```python
from build123d import *

# Parameters (mm, degrees)
SKETCH1_W                = 130
SKETCH1_H                = 80
BOSS_EXTRUDE1_DEPTH      = 2
CUT_EXTRUDE_THIN1_DEPTH  = 3.2
BOSS_EXTRUDE2_DEPTH      = 10
BOSS_EXTRUDE2_DEPTH_BACK = 15
SKETCH5_R                = 1.5
BOSS_EXTRUDE3_DEPTH      = 10
BOSS_EXTRUDE3_DEPTH_BACK = 12
SKETCH6_R                = 2
SKETCH9_W                = 5
SKETCH9_H                = 50
BOSS_EXTRUDE5_DEPTH      = 10.5
SKETCH11_R               = 1.5
CUT_EXTRUDE1_DEPTH       = 7.5


with BuildPart() as part:
    # Sketch1 → Boss-Extrude1 (new body)
    with BuildSketch(Plane.XY):
        with Locations((65, 40)):
            Rectangle(SKETCH1_W, SKETCH1_H)
    extrude(amount=BOSS_EXTRUDE1_DEPTH)

    # Sketch2 → Cut-Extrude-Thin1 (cut)
    with BuildSketch(Plane.XY.offset(2)):
        with BuildLine():
            Line((49.817075189, 61.102777477), (79.817075189, 57.949650419))
            ThreePointArc((79.817075189, 57.949650419), (81.8288026, 55.594220253), (79.581886147, 53.461976154))
            Line((79.581886147, 53.461976154), (49.581886147, 53.461976154))
            ThreePointArc((49.581886147, 53.461976154), (43.839766322, 48.012907902), (48.980847483, 41.993475256))
            Line((48.980847483, 41.993475256), (68.980847483, 39.89139055))
            ThreePointArc((68.980847483, 39.89139055), (70.992574894, 37.535960384), (68.745658441, 35.403716286))
            Line((68.745658441, 35.403716286), (48.745658441, 35.403716286))
            ThreePointArc((48.745658441, 35.403716286), (43.003538616, 29.954648034), (48.144619777, 23.935215387))
            Line((48.144619777, 23.935215387), (102.144619777, 18.259586683))
            Line((102.144619777, 18.259586683), (102.510469398, 21.740413317))
            Line((102.510469398, 21.740413317), (48.510469398, 27.416042021))
            ThreePointArc((48.510469398, 27.416042021), (46.498741988, 29.771472187), (48.745658441, 31.903716286))
            Line((48.745658441, 31.903716286), (68.745658441, 31.903716286))
            ThreePointArc((68.745658441, 31.903716286), (74.487778266, 37.352784537), (69.346697105, 43.372217184))
            Line((69.346697105, 43.372217184), (49.346697105, 45.47430189))
            ThreePointArc((49.346697105, 45.47430189), (47.334969694, 47.829732056), (49.581886147, 49.961976154))
            Line((49.581886147, 49.961976154), (79.581886147, 49.961976154))
            ThreePointArc((79.581886147, 49.961976154), (85.324005972, 55.411044406), (80.182924811, 61.430477052))
            Line((80.182924811, 61.430477052), (50.182924811, 64.58360411))
            Line((50.182924811, 64.58360411), (49.817075189, 61.102777477))
        make_face()
    extrude(amount=-CUT_EXTRUDE_THIN1_DEPTH, mode=Mode.SUBTRACT)

    # Sketch5 → Boss-Extrude2 (add, two sides: drawn at the far end of the back side and taken through both)
    with BuildSketch(Plane(origin=(0, 0, 0), x_dir=(-1, 0, 0), z_dir=(0, 0, -1)).offset(-BOSS_EXTRUDE2_DEPTH_BACK)):
        with Locations((-115, 10)):
            Circle(SKETCH5_R)
    extrude(amount=BOSS_EXTRUDE2_DEPTH + BOSS_EXTRUDE2_DEPTH_BACK)

    # Sketch6 → Boss-Extrude3 (add, two sides: drawn at the far end of the back side and taken through both)
    with BuildSketch(Plane(origin=(0, 0, 0), x_dir=(-1, 0, 0), z_dir=(0, 0, -1)).offset(-BOSS_EXTRUDE3_DEPTH_BACK)):
        with Locations((-13.162577251, 8.793885197)):
            Circle(SKETCH6_R)
    extrude(amount=BOSS_EXTRUDE3_DEPTH + BOSS_EXTRUDE3_DEPTH_BACK)

    # Sketch9 → Boss-Extrude5 (add)
    with BuildSketch(Plane.XY.offset(2)):
        with Locations((96.5, 40)):
            Rectangle(SKETCH9_W, SKETCH9_H)
    extrude(amount=-BOSS_EXTRUDE5_DEPTH)

    # Sketch11 → Cut-Extrude1 (cut)
    with BuildSketch(Plane.ZY.offset(-94)):
        with Locations((-4.25, 55.711976154)):
            Circle(SKETCH11_R)
        with Locations((-4.25, 37.653716286)):
            Circle(SKETCH11_R)
        with Locations((-4.25, 22.837814352)):
            Circle(SKETCH11_R)
    extrude(amount=-CUT_EXTRUDE1_DEPTH, mode=Mode.SUBTRACT)


solid = part.part
```
Geometry check sheet. Reference: the model listing, model coordinates, mm. A direction names the side the tool comes from. Coordinates: 2 decimals unless noted, no trailing zeros. Loops run counter-clockwise (first coordinate to the right, second up) from the corner with the lowest first, then second, coordinate; pieces in that order, holes last.
Item 1: Release check for a two-part mould opening along X. For faces 1 (the face through (12.24, 7.02, 7.07)), 2 (the face through (96.465, 21.373, -4.575)) record: released by +X, released by -X, zero draft, split by the parting line, or undercut.
Item 2: Sectioned sample at D-D, the plane y = 74. Record the boundary of the cut face in (x, z), then the cut area to 3 significant figures.
Item 3: Sectioned sample at A-A, the plane x = 78. Record the boundary of the cut face in (y, z).
Item 4: Access from +Z, -Z, +X, -X, +Y, -Y to the whole of each face (thin tool, end or side, straight path). Record for faces 3 (the face through (43.847, 48.135, 1.014)), 4 (the face through (116.5, 10.07, 8.59)), 5 (the face through (13, 9, 12)), 6 (the face through (12.24, 7.02, -4.93)), 7 (the face through (96, 15, -4)).
Item 5: Sectioned sample at C-C, the plane x = 115. Record the boundary of the cut face in (y, z).
Item 6: Thickness scan on line 1 (Y direction, x = 95.2, z = -4.25); line 2 (Z direction, x = 91, y = 30); line 3 (X direction, y = 40.5, z = -6.25). Record the ranges inside material, lowest first.
Item 7: Go/stop test with flat-tipped pins: pin 1 Ø24 at (x, y) = (73, 48.5) entering from -Z; pin 2 Ø2.5 at (x, z) = (96.5, -3) entering from -Y; pin 3 Ø11.5 at (y, z) = (51, -6) entering from -X. Record where each tip stops, or that it passes through.
Item 8: Sectioned sample at B-B, the plane z = -4.25. Record the boundary of the cut face in (x, y).
Check result:
1. face 1: undercut
1. face 2: zero draft
2. outline: (0, 0) - (130, 0) - (130, 2) - (0, 2) - close
2. area: 260 mm2
3. outline: (0, 0) - (20.8, 0) - (20.8, 2) - (0, 2) - close; (24.32, 0) - (49.96, 0) - (49.96, 2) - (24.32, 2) - close; (53.46, 0) - (58.14, 0) - (58.14, 2) - (53.46, 2) - close; (61.66, 0) - (80, 0) - (80, 2) - (61.66, 2) - close
4. face 3: +Z, -Z
4. face 4: +Z
4. face 5: +Z, -X, +Y, -Y
4. face 6: -Z
4. face 7: -Z, +X, -X, -Y
5. outline: (0, 0) - (8.5, 0) - (8.5, -10) - (11.5, -10) - (11.5, 0) - (80, 0) - (80, 2) - (11.5, 2) - (11.5, 15) - (8.5, 15) - (8.5, 2) - (0, 2) - close
6. line 1: y = 15 to 21.34, 24.34 to 36.15, 39.15 to 54.21, 57.21 to 65
6. line 2: z = 0 to 2
6. line 3: x = 94 to 99
7. pin 1: stops at z = 0
7. pin 2: stops at y = 15
7. pin 3: stops at x = 94
8. outline: circle Ø4 at (13.16, 8.79); (94, 15) - (99, 15) - (99, 21.34) - (94, 21.34) - close; (94, 24.34) - (99, 24.34) - (99, 36.15) - (94, 36.15) - close; (94, 39.15) - (99, 39.15) - (99, 54.21) - (94, 54.21) - close; (94, 57.21) - (99, 57.21) - (99, 65) - (94, 65) - close; circle Ø3 at (115, 10)
